Check sheet for the modelled part. Datum: model origin and axes. Units: mm. A direction names the side the tool comes from. Coordinates: 2 decimals unless noted, no trailing zeros. Order: outer loops, then holes, each group sorted by start corner. A loop starts at its lowest first (then second) coordinate and runs counter-clockwise, first axis right, second up.
1. Cross-section at B-B (x = 36.5). Enter the section's corners in (y, z), then the cut area to 3 significant figures.
2. Draft check along X on faces 1 (the flat face through (52, 8.6, 47)), 2 (the cylindrical face through (50.9, 3.7, 49.2)). Enter one of: released by +X, released by -X, zero draft, split by the parting line, or undercut.
3. Cross-section at D-D (y = 1.25). Enter the section's corners in (x, z).
4. Cross-section at A-A (z = 30). Enter the section's corners in (x, y).
5. Thickness scan on line 1 (X direction, y = 4.9, z = 10); line 2 (X direction, y = 0.65, z = 30); line 3 (Z direction, x = 51.5, y = 4.4) (3 decimals). Record the ranges inside material, lowest first.
6. Gauge pin test, flat ends, axial feed: pin 1 Ø4 at (y, z) = (7, 11.5) entering from +X; pin 2 Ø2.5 at (x, z) = (51.5, 50) entering from +Y; pin 3 Ø2.5 at (x, z) = (3.67, 3.39) entering from +Y; pin 4 Ø4 at (x, z) = (51.5, 10) entering from +Y. Record the tip position at first contact, or that the pin passes through.
7. Set-up check for faces 3 (the cylindrical face through (24.94, 1.23, 14.92)), 4 (the flat face through (13, 3, 50)), 5 (the cylindrical face through (62.717, 1.479, 57.496)): record each of +Z, -Z, +X, -X, +Y, -Y from which the full face is reachable in a straight line by a thin tool's end or side.
8. Cross-section at C-C (y = 6.25). Enter the section's corners in (x, z).
```python
from build123d import *

# Parameters (mm, degrees)
SKETCH2_W           = 65
SKETCH2_H           = 60
SKETCH2_R           = 1.65
BOSS_EXTRUDE1_DEPTH = 3
SKETCH3_R           = 24
BOSS_EXTRUDE2_DEPTH = 1.5
SKETCH5_R           = 19
CUT_EXTRUDE1_DEPTH  = 2.5
SKETCH6_R           = 2.5
CUT_EXTRUDE2_DEPTH  = 89.573415876
SKETCH7_R           = 3.2
SKETCH7_R_2         = 1.6
BOSS_EXTRUDE3_DEPTH = 5.6
FILLET1_R           = 1


with BuildPart() as part:
    # Sketch2 → Boss-Extrude1 (new body)
    with BuildSketch(Plane(origin=(0, 0, 0), x_dir=(1, 0, 0), z_dir=(0, 1, 0))):
        with Locations((32.5, -30)):
            Rectangle(SKETCH2_W, SKETCH2_H)
        with Locations(Location((3.674017223, -3.391400514, 0), (0, 0, 270))):
            Circle(SKETCH2_R, mode=Mode.SUBTRACT)
        with Locations(Location((61.325982777, -3.391400514, 0), (0, 0, 270))):
            Circle(SKETCH2_R, mode=Mode.SUBTRACT)
        with Locations(Location((61.325982777, -56.608599486, 0), (0, 0, 270))):
            Circle(SKETCH2_R, mode=Mode.SUBTRACT)
        with Locations(Location((3.674017223, -56.608599486, 0), (0, 0, 270))):
            Circle(SKETCH2_R, mode=Mode.SUBTRACT)
    extrude(amount=BOSS_EXTRUDE1_DEPTH)

    # Sketch3 → Boss-Extrude2 (add)
    with BuildSketch(Plane(origin=(0, 3, 0), x_dir=(1, 0, 0), z_dir=(0, 1, 0))):
        with Locations(Location((36.5, -30, 0), (0, 0, 270))):
            Circle(SKETCH3_R)
    extrude(amount=BOSS_EXTRUDE2_DEPTH)

    # Sketch5 → Cut-Extrude1 (cut)
    with BuildSketch(Plane(origin=(0, 0, 0), x_dir=(1, 0, 0), z_dir=(0, 1, 0))):
        with Locations(Location((36.5, -30, 0), (0, 0, 270))):
            Circle(SKETCH5_R)
    extrude(amount=CUT_EXTRUDE1_DEPTH, mode=Mode.SUBTRACT)

    # Sketch6 → Cut-Extrude2 (cut, through all)
    with BuildSketch(Plane(origin=(0, 4.5, 0), x_dir=(1, 0, 0), z_dir=(0, 1, 0))):
        with Locations(Location((36.5, -30, 0), (0, 0, 270))):
            Circle(SKETCH6_R)
    extrude(amount=-CUT_EXTRUDE2_DEPTH, mode=Mode.SUBTRACT)

    # Sketch7 → Boss-Extrude3 (add)
    # profile 1 of 4: a face of its own
    with BuildSketch(Plane(origin=(0, 3, 0), x_dir=(1, 0, 0), z_dir=(0, 1, 0))):
        with Locations(Location((13.5, -10, 0), (0, 0, 270))):
            Circle(SKETCH7_R)
        with Locations(Location((13.5, -10, 0), (0, 0, 270))):
            Circle(SKETCH7_R_2, mode=Mode.SUBTRACT)
    # profile 2 of 4: a face of its own
    with BuildSketch(Plane(origin=(0, 3, 0), x_dir=(1, 0, 0), z_dir=(0, 1, 0))):
        with Locations(Location((13.5, -50, 0), (0, 0, 270))):
            Circle(SKETCH7_R)
        with Locations(Location((13.5, -50, 0), (0, 0, 270))):
            Circle(SKETCH7_R_2, mode=Mode.SUBTRACT)
    # profile 3 of 4: a face of its own
    with BuildSketch(Plane(origin=(0, 3, 0), x_dir=(1, 0, 0), z_dir=(0, 1, 0))):
        with Locations(Location((51.5, -10, 0), (0, 0, 164.861138608))):
            Circle(SKETCH7_R)
        with Locations(Location((51.5, -10, 0), (0, 0, 183.258299887))):
            Circle(SKETCH7_R_2, mode=Mode.SUBTRACT)
    # profile 4 of 4: a face of its own
    with BuildSketch(Plane(origin=(0, 3, 0), x_dir=(1, 0, 0), z_dir=(0, 1, 0))):
        with Locations(Location((51.5, -50, 0), (0, 0, 58.600933899))):
            Circle(SKETCH7_R)
        with Locations(Location((51.5, -50, 0), (0, 0, 76.998095179))):
            Circle(SKETCH7_R_2, mode=Mode.SUBTRACT)
    extrude(amount=BOSS_EXTRUDE3_DEPTH)

    # Fillet1
    fillet1_edges = [part.edges().sort_by_distance(p)[0] for p in [
        (13.5, 8.6, 48.4),
        (53.097413516, 8.6, 9.909060137),
        (51.140026484, 8.6, 51.558980137),
        (13.5, 8.6, 8.4),
    ]]
    fillet(fillet1_edges, radius=FILLET1_R)


solid = part.part
```
Data:
1. outline: (0, 0) - (3, 0) - (3, 6) - (4.5, 6) - (4.5, 27.5) - (2.5, 27.5) - (2.5, 11) - (0, 11) - close; (0, 49) - (2.5, 49) - (2.5, 32.5) - (4.5, 32.5) - (4.5, 54) - (3, 54) - (3, 60) - (0, 60) - close
1. area: 147 mm2
2. face 1: zero draft
2. face 2: undercut
3. outline: (0, 0) - (65, 0) - (65, 60) - (0, 60) - close; hole circle Ø3.3 at (3.67, 3.39); hole circle Ø3.3 at (3.67, 56.61); hole circle Ø38 at (36.5, 30); hole circle Ø3.3 at (61.33, 3.39); hole circle Ø3.3 at (61.33, 56.61)
4. outline: (0, 0) - (17.5, 0) - (17.5, 2.5) - (34, 2.5) - (34, 4.5) - (12.5, 4.5) - (12.5, 3) - (0, 3) - close; (39, 2.5) - (55.5, 2.5) - (55.5, 0) - (65, 0) - (65, 3) - (60.5, 3) - (60.5, 4.5) - (39, 4.5) - close
5. line 1: x = 10.3 to 11.9, 15.1 to 16.7, 48.3 to 49.9, 53.1 to 54.7
5. line 2: x = 0 to 17.5, 55.5 to 65
5. line 3: z = 6.8 to 8.4, 11.265 to 48.735, 51.6 to 53.2
6. pin 1: stops at x = 54.7
6. pin 2: stops at y = 4.5
6. pin 3: passes through
6. pin 4: stops at y = 8.4
7. face 3: -Y
7. face 4: +Y
7. face 5: +Y, -Y
8. outline: circle Ø6.4 at (13.5, 10); circle Ø6.4 at (13.5, 50); circle Ø6.4 at (51.5, 10); circle Ø6.4 at (51.5, 50); hole circle Ø3.2 at (13.5, 10); hole circle Ø3.2 at (13.5, 50); hole circle Ø3.2 at (51.5, 10); hole circle Ø3.2 at (51.5, 50)
